Could you check a few things on this model? Use its own coordinates, in mm. Round coordinates to 2 decimals unless told otherwise and drop trailing zeros. Write each loop counter-clockwise with the first axis right and the second up, starting at its lowest first coordinate (ties: lowest second). Pieces come first, ordered by that corner, then holes. Notation, with made-up numbers: M -4,9.5 L 39,9.5 A26 ccw 39,43.5 Z; hole C 59.25,8.25 d6. An arc over 180 degrees is marked long. One line per item, written item: value. Start each with the question number.
(1) Thinking about a two-plate mould opening in Y: for faces 1 (the face through (26, -113, 28)), 2 (the face through (20, 7, 28)), 3 (the face through (13, 141.034, 28)), 4 (the face through (20, -228, 28)), which applies, released by +Y, released by -Y, zero draft, split by the parting line, or undercut?
(2) I'm going to push flat-ended pins straight in: pin 1 Ø20.5 at (y, z) = (6, 36.5) entering from +X; pin 2 Ø5 at (y, z) = (126.03, 27.84) entering from -X. Where does each tip first touch, or does it pass through?
(3) I want a section at A-A on y = -29.5. Please give me the cut outline in (x, z).
(4) If I drill on L1, parallel to Y at x = 24.5, z = 18; L2, parallel to Y at x = 23, z = 43; L3, parallel to Y at x = 13.25, z = 11.5, over which ranges is the centre line in solid material (lowest first)?
```python
from build123d import *

# Parameters (mm, degrees)
F0_W     = 500
F0_H     = 41
F0_R     = 3
F0_R_2   = 3.25
F1_DEPTH = 26
F2_W     = 6
F2_H     = 205
F3_DEPTH = 41


with BuildPart() as f1:
    # F0 (on Right) → F1 (new body)
    with BuildSketch(Plane.YZ):
        with Locations((-108.96641, 27.840261)):
            Rectangle(F0_W, F0_H)
        with Locations((-343.96641, 12.840261)):
            Circle(F0_R, mode=Mode.SUBTRACT)
        with Locations((-343.96641, 27.840261)):
            Circle(F0_R_2, mode=Mode.SUBTRACT)
        with Locations((-108.96641, 12.840261)):
            Circle(F0_R, mode=Mode.SUBTRACT)
        with Locations((126.03359, 12.840261)):
            Circle(F0_R, mode=Mode.SUBTRACT)
        with Locations((-343.96641, 42.840261)):
            Circle(F0_R, mode=Mode.SUBTRACT)
        with Locations((-108.96641, 27.840261)):
            Circle(F0_R_2, mode=Mode.SUBTRACT)
        with Locations((126.03359, 27.840261)):
            Circle(F0_R_2, mode=Mode.SUBTRACT)
        with Locations((-108.96641, 42.840261)):
            Circle(F0_R, mode=Mode.SUBTRACT)
        with Locations((126.03359, 42.840261)):
            Circle(F0_R, mode=Mode.SUBTRACT)
    extrude(amount=F1_DEPTH)

    # F2 (on face) → F3 (cut, through all)
    with BuildSketch(Plane.XY.offset(48.340261)):
        with Locations((23, -226.46641)):
            Rectangle(F2_W, F2_H)
        with Locations((23, 8.53359)):
            Rectangle(F2_W, F2_H)
    extrude(amount=-F3_DEPTH, mode=Mode.SUBTRACT)


solid = f1.part
```
Found:
1. face 1: zero draft
1. face 2: undercut
1. face 3: released by +Y
1. face 4: undercut
2. pin 1: stops at x = 20
2. pin 2: passes through
3. outline: M 0,7.34 L 20,7.34 L 20,48.34 L 0,48.34 Z
4. L1: y = -358.97 to -328.97, -123.97 to -93.97, 111.03 to 141.03
4. L2: y = -358.97 to -346.96, -340.97 to -328.97, -123.97 to -111.96, -105.97 to -93.97, 111.03 to 123.04, 129.03 to 141.03
4. L3: y = -358.97 to -346.65, -341.28 to -111.65, -106.28 to 123.35, 128.72 to 141.03
